For this review, take the finished solid that the model builds, in its own axes (mm). Face numbers are marked on the shaded views. A direction names the side the tool comes from. Coordinates: 2 decimals unless noted, no trailing zeros. Order: outer loops, then holes, each group sorted by start corner. A loop starts at its lowest first (then second) coordinate and runs counter-clockwise, first axis right, second up. Notation, with made-up numbers: (-37, 19) -> (10, 19) arc R27 ccw to (10, 50) -> close; hole circle Ø1 at (-38.75, 21.25). An arc over 180 degrees is marked (long way). Return JSON: item names as keys, results as strings. Group by question number.
Item 1: Take a section at D-D (z = 179). Write out the cut boundary in (x, y), then the cut area to 3 significant figures.
Item 2: Insertion check: pin 1 (5 mm diameter, centred on x = -30, z = 185, fed in from -Y); pin 2 (2.5 mm diameter, centred on x = -10, z = 185, fed in from +Y); pin 3 (6 mm diameter, centred on x = -32.5, y = 6.5, fed in from +Z); pin 4 (4 mm diameter, centred on x = -24, z = 186.5, fed in from +Y). Each pin has a flat end and moves straight along its axis. Give the tip position at first contact, or say it passes through.
Item 3: Take a section at B-B (z = 185). Write out the cut boundary in (x, y), then the cut area to 4 significant figures.
Item 4: Take a section at C-C (y = -6.5). Write out the cut boundary in (x, z).
Item 5: Take a section at A-A (x = -30). Write out the cut boundary in (y, z).
Item 6: Draft analysis for pull direction X (two halves, no side actions). For the marked faces 4, 5 and 6, state which applies: +X half, -X half, draft (parallel to the pull), parting line (faces both ways), or undercut.
Item 7: For line 1 along X through (y, z) = (2.8, 185); line 2 along X through (y, z) = (-2.5, 192.75); line 3 along X through (y, z) = (3, 185.75), list the stretches that pass through material, from the lowest coordinate up.
Item 8: Machinability: for the marked faces 1, 2 and 3, which of the approach directions +Z, -Z, +X, -X, +Y, -Y give a long, thin tool a straight path to every point of the face, cutting with its end or side? Answer none if there is none.
```python
from build123d import *

# Parameters (mm, degrees)
CROQUIS1_R              = 2.25
SALIENTE_EXTRUIR1_DEPTH = 4.5
CROQUIS3_W              = 5
CROQUIS3_H              = 20
SALIENTE_EXTRUIR3_DEPTH = 5.5
CROQUIS4_W              = 5
CROQUIS4_H              = 20
SALIENTE_EXTRUIR4_DEPTH = 10


with BuildPart() as part:
    # Croquis1 → Saliente-Extruir1 (new body)
    with BuildSketch(Plane(origin=(0, 0, 0), x_dir=(1, 0, 0), z_dir=(0, 1, 0))):
        Polygon((-35, -175), (-45, -175), (-45, -195), (-35, -195), (-5, -195), (5, -195), (5, -175), (-5, -175), align=None)
        with Locations(Location((-30, -185, 0), (0, 0, 270))):
            Circle(CROQUIS1_R, mode=Mode.SUBTRACT)
        with Locations(Location((-10, -185, 0), (0, 0, 270))):
            Circle(CROQUIS1_R, mode=Mode.SUBTRACT)
    extrude(amount=SALIENTE_EXTRUIR1_DEPTH)

    # Croquis3 → Saliente-Extruir3 (add)
    with BuildSketch(Plane(origin=(0, 4.5, 0), x_dir=(1, 0, 0), z_dir=(0, 1, 0))):
        with Locations((2.5, -185)):
            Rectangle(CROQUIS3_W, CROQUIS3_H)
        with Locations((-42.5, -185)):
            Rectangle(CROQUIS3_W, CROQUIS3_H)
    extrude(amount=SALIENTE_EXTRUIR3_DEPTH)

    # Croquis4 → Saliente-Extruir4 (add)
    with BuildSketch(Plane.XZ):
        with Locations((2.5, 185)):
            Rectangle(CROQUIS4_W, CROQUIS4_H)
        Polygon((-40, 175), (-40, 195), (-45, 195), (-45, 175), (-40.824678474, 175), align=None)
    extrude(amount=SALIENTE_EXTRUIR4_DEPTH)


solid = part.part
```
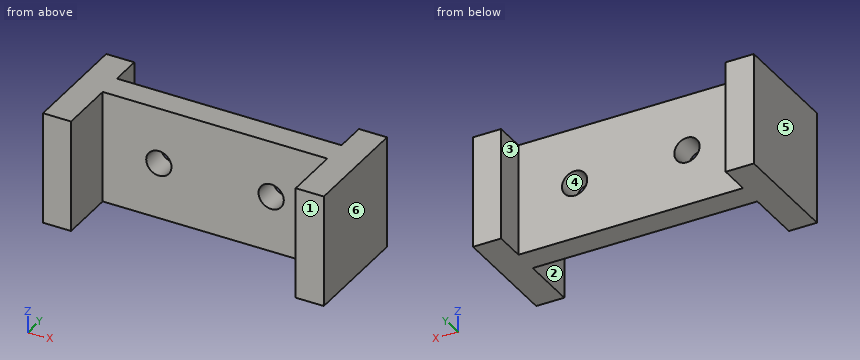
Findings below:
{
 "1": {"outline": "(-45, -10) -> (-40, -10) -> (-40, 0) -> (0, 0) -> (0, -10) -> (5, -10) -> (5, 10) -> (0, 10) -> (0, 4.5) -> (-40, 4.5) -> (-40, 10) -> (-45, 10) -> close", "area": "380 mm2"},
 "2": {"pin 1": "stops at y = 0", "pin 2": "passes through", "pin 3": "stops at z = 195", "pin 4": "stops at y = 4.5"},
 "3": {"outline": "(-45, -10) -> (-40, -10) -> (-40, 0) -> (-32.25, 0) -> (-32.25, 4.5) -> (-40, 4.5) -> (-40, 10) -> (-45, 10) -> close; (-27.75, 0) -> (-12.25, 0) -> (-12.25, 4.5) -> (-27.75, 4.5) -> close; (-7.75, 0) -> (0, 0) -> (0, -10) -> (5, -10) -> (5, 10) -> (0, 10) -> (0, 4.5) -> (-7.75, 4.5) -> close", "area": "339.5 mm2"},
 "4": {"outline": "(-45, 175) -> (-40, 175) -> (-40, 195) -> (-45, 195) -> close; (0, 175) -> (5, 175) -> (5, 195) -> (0, 195) -> close"},
 "5": {"outline": "(0, 175) -> (4.5, 175) -> (4.5, 182.75) -> (0, 182.75) -> close; (0, 187.25) -> (4.5, 187.25) -> (4.5, 195) -> (0, 195) -> close"},
 "6": {"face 4": "undercut", "face 5": "-X half", "face 6": "+X half"},
 "7": {"line 1": "x = -45 to -32.25, -27.75 to -12.25, -7.75 to 5", "line 2": "x = -45 to -40, 0 to 5", "line 3": "x = -45 to -32.12, -27.88 to -12.12, -7.88 to 5"},
 "8": {"face 1": "+Z, -Z, +X, -X, -Y", "face 2": "+Z, -Z, -Y", "face 3": "+Z, -Z, +Y"}
}
